Could you check a few things on this model? Use its own coordinates, in mm. Face numbers are marked on the shaded views. A direction names the side the tool comes from. Coordinates: 2 decimals unless noted, no trailing zeros. Write each loop counter-clockwise with the first axis right and the second up, starting at its lowest first coordinate (ties: lowest second). Pieces come first, ordered by that corner, then holes.
Item 1: I want a section at A-A on x = -63.5. Please give me the cut outline in (y, z) (1 decimal), then the cut area to 3 significant figures.
Item 2: I want a section at B-B on y = -47. Please give me the cut outline in (x, z) (3 decimals).
Item 3: Which directions (+Z, -Z, +X, -X, +Y, -Y) give clear straight access to the entire face, cutting with the end or side of a thin tool? Please do the marked faces 4, 5, 6, 7 and 8.
Item 4: If I drill on probe 1 along Z at (x, y) = (-63.5, -24.5); probe 2 along X at (y, z) = (-45, 32.5) (3 decimals); probe 3 along Z at (x, y) = (-6, -31), over which ranges is the centre line in solid material (lowest first)?
Item 5: Thinking about a two-plate mould opening in X: for the marked faces 1, 2 and 3, which applies, +X half, -X half, draft (parallel to the pull), parting line (faces both ways), or undercut?
Item 6: For P1, Ø24, axis at y = -52.5, z = 30.5, coming from the +X side (3 decimals); P2, Ø19, axis at x = -56.5, z = 36, coming from the -Y side; P3, Ø23, axis at x = -116, z = 31, coming from the -Y side, each with a flat end and sliding along its axis, tell me the tip position at first contact or that it passes through.
Item 7: I want a section at D-D on y = -26.5. Please give me the cut outline in (x, z) (1 decimal).
from build123d import *

# Parameters (mm, degrees)
F0_W     = 31.75
F0_H     = 31.75
F1_DEPTH = 31.75
F2_DEPTH = 92.075
F3_DEPTH = 53.975
F0_H_2   = 88.9
F4_DEPTH = 73.025
F5_SCALE = 0.5


with BuildPart() as f1:
    # F0 (on Front) → F1 (new body)
    with BuildSketch(Plane.XZ):
        Polygon((-69.85, 84.0967045993), (-127, 84.0967045993), (-127, 33.2967045993), (-85.725, 33.2967045993), (-85.725, -17.5032954007), (-127, -17.5032954007), (-127, -68.3032954007), (-69.85, -68.3032954007), (-69.85, -36.5532954007), (-69.85, 52.3467045993), align=None)
        with Locations((-53.975, 68.2217045993)):
            Rectangle(F0_W, F0_H)
        with BuildLine():
            Line((0, 84.0967045993), (-38.1, 84.0967045993))
            Line((-38.1, 84.0967045993), (-38.1, 52.3467045993))
            Line((-38.1, 52.3467045993), (-38.1, -36.5532954007))
            Line((-38.1, -36.5532954007), (-38.1, -68.3032954007))
            Line((-38.1, -68.3032954007), (0, -68.3032954007))
            Line((0, -68.3032954007), (0, -15.875))
            Line((0, -15.875), (0, -7.9782954007))
            ThreePointArc((0, -7.9782954007), (-15.875, 7.8967045993), (0, 23.7717045993))
            Line((0, 23.7717045993), (0, 84.0967045993))
        make_face()
        with BuildLine():
            Line((38.1, 84.0967045993), (0, 84.0967045993))
            Line((0, 84.0967045993), (0, 23.7717045993))
            ThreePointArc((0, 23.7717045993), (11.2253201513, 19.1220247506), (15.875, 7.8967045993))
            ThreePointArc((15.875, 7.8967045993), (11.2253201513, -3.3286155521), (0, -7.9782954007))
            Line((0, -7.9782954007), (0, -15.875))
            Line((0, -15.875), (0, -68.3032954007))
            Line((0, -68.3032954007), (38.1, -68.3032954007))
            Line((38.1, -68.3032954007), (38.1, -36.5532954007))
            Line((38.1, -36.5532954007), (38.1, 52.3467045993))
            Line((38.1, 52.3467045993), (38.1, 84.0967045993))
        make_face()
        with Locations((-53.975, -52.4282954007)):
            Rectangle(F0_W, F0_H)
        with Locations((53.975, 68.2217045993)):
            Rectangle(F0_W, F0_H)
        Polygon((127, 84.0967045993), (69.85, 84.0967045993), (69.85, 52.3467045993), (69.85, -36.5532954007), (69.85, -68.3032954007), (127, -68.3032954007), (127, -17.5032954007), (85.725, -17.5032954007), (85.725, 33.2967045993), (127, 33.2967045993), align=None)
        with Locations((53.975, -52.4282954007)):
            Rectangle(F0_W, F0_H)
    extrude(amount=F1_DEPTH)

    # F0 (on Front) → F2 (join)
    with BuildSketch(Plane.XZ):
        with Locations((-53.975, 68.2217045993)):
            Rectangle(F0_W, F0_H)
        with Locations((-53.975, -52.4282954007)):
            Rectangle(F0_W, F0_H)
        with Locations((53.975, -52.4282954007)):
            Rectangle(F0_W, F0_H)
        with Locations((53.975, 68.2217045993)):
            Rectangle(F0_W, F0_H)
    extrude(amount=F2_DEPTH)

    # F0 (on Front) → F3 (join)
    with BuildSketch(Plane.XZ):
        with BuildLine():
            Line((0, 84.0967045993), (-38.1, 84.0967045993))
            Line((-38.1, 84.0967045993), (-38.1, 52.3467045993))
            Line((-38.1, 52.3467045993), (-38.1, -36.5532954007))
            Line((-38.1, -36.5532954007), (-38.1, -68.3032954007))
            Line((-38.1, -68.3032954007), (0, -68.3032954007))
            Line((0, -68.3032954007), (0, -15.875))
            Line((0, -15.875), (0, -7.9782954007))
            ThreePointArc((0, -7.9782954007), (-15.875, 7.8967045993), (0, 23.7717045993))
            Line((0, 23.7717045993), (0, 84.0967045993))
        make_face()
        with BuildLine():
            Line((38.1, 84.0967045993), (0, 84.0967045993))
            Line((0, 84.0967045993), (0, 23.7717045993))
            ThreePointArc((0, 23.7717045993), (11.2253201513, 19.1220247506), (15.875, 7.8967045993))
            ThreePointArc((15.875, 7.8967045993), (11.2253201513, -3.3286155521), (0, -7.9782954007))
            Line((0, -7.9782954007), (0, -15.875))
            Line((0, -15.875), (0, -68.3032954007))
            Line((0, -68.3032954007), (38.1, -68.3032954007))
            Line((38.1, -68.3032954007), (38.1, -36.5532954007))
            Line((38.1, -36.5532954007), (38.1, 52.3467045993))
            Line((38.1, 52.3467045993), (38.1, 84.0967045993))
        make_face()
    extrude(amount=F3_DEPTH)

    # F0 (on Front) → F4 (join)
    with BuildSketch(Plane.XZ):
        with Locations((-53.975, 7.8967045993)):
            Rectangle(F0_W, F0_H_2)
        with Locations((53.975, 7.8967045993)):
            Rectangle(F0_W, F0_H_2)
    extrude(amount=F4_DEPTH)


with BuildPart() as f1_1:
    # F5: moved
    add(f1.part.scale(F5_SCALE).moved(Location((-63.5, -15.875, 42.0483522996))))


solid = f1_1.part
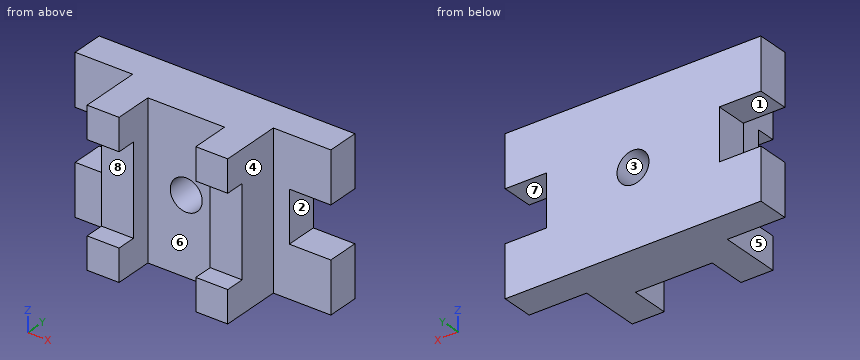
Response values:
1. outline: (-42.9, 7.9) - (-15.9, 7.9) - (-15.9, 38.1) - (-42.9, 38.1) - close; (-42.9, 53.9) - (-15.9, 53.9) - (-15.9, 84.1) - (-42.9, 84.1) - close
1. area: 1,630 mm2
2. outline: (-98.425, 7.897) - (-82.55, 7.897) - (-82.55, 84.097) - (-98.425, 84.097) - close; (-44.45, 7.897) - (-28.575, 7.897) - (-28.575, 84.097) - (-44.45, 84.097) - close
3. face 4: +Z, -Z, +X, -Y
3. face 5: +Z, -Z, -X, -Y
3. face 6: +Z, -Z, -Y
3. face 7: +X, +Y, -Y
3. face 8: +X, -X, -Y
4. probe 1: z = 7.9 to 38.06, 53.93 to 84.1
4. probe 2: x = -98.425 to -82.55, -44.45 to -28.575
4. probe 3: z = 7.9 to 33.3, 58.7 to 84.1
5. face 1: draft
5. face 2: +X half
5. face 3: undercut
6. P1: stops at x = -28.575
6. P2: stops at y = -42.86
6. P3: stops at y = -31.75
7. outline: (-127, 7.9) - (0, 7.9) - (0, 33.3) - (-20.6, 33.3) - (-20.6, 58.7) - (0, 58.7) - (0, 84.1) - (-127, 84.1) - (-127, 58.7) - (-106.4, 58.7) - (-106.4, 33.3) - (-127, 33.3) - close; hole circle Ø15.9 at (-63.5, 46)
